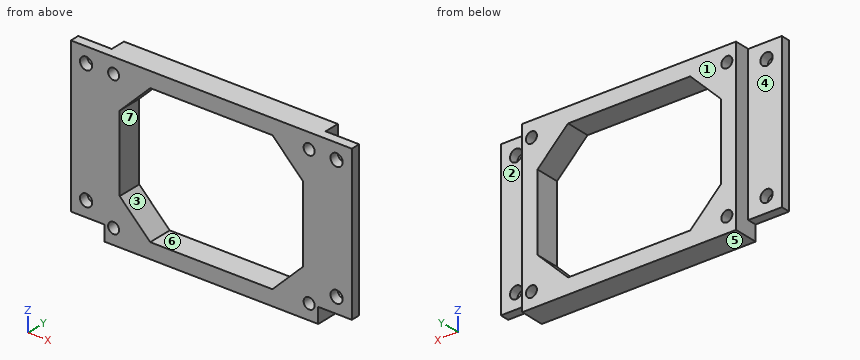
```python
from build123d import *

# Parameters (mm, degrees)
SKETCH1_W                = 70
SKETCH1_H                = 50
BOSS_EXTRUDE1_DEPTH      = 5
SKETCH2_W                = 92
SKETCH2_H                = 50
BOSS_EXTRUDE2_DEPTH      = 3
M3_CLEARANCE_HOLE1_D     = 4
M3_CLEARANCE_HOLE1_DEPTH = 10
M3_CLEARANCE_HOLE1_TIP   = 1.201721238
SKETCH9_W                = 70
SKETCH9_H                = 8
BOSS_EXTRUDE3_DEPTH      = 5
M3_CLEARANCE_HOLE3_D     = 3.6
M3_CLEARANCE_HOLE3_DEPTH = 10
M3_CLEARANCE_HOLE3_TIP   = 1.081549114
CUT_EXTRUDE1_DEPTH       = 56.497747702


with BuildPart() as part:
    # Sketch1 → Boss-Extrude1 (new body)
    with BuildSketch(Plane(origin=(0, 0, 0), x_dir=(1, 0, 0), z_dir=(0, 1, 0))):
        Rectangle(SKETCH1_W, SKETCH1_H)
    extrude(amount=BOSS_EXTRUDE1_DEPTH)

    # Sketch2 → Boss-Extrude2 (add)
    with BuildSketch(Plane.XZ):
        Rectangle(SKETCH2_W, SKETCH2_H)
    extrude(amount=BOSS_EXTRUDE2_DEPTH)

    # M3 Clearance Hole1
    with Locations(Plane(origin=(0, 0, 0), x_dir=(1, 0, 0), z_dir=(0, 1, 0))):
        with Locations((-41, 20), (-41, -20), (41, 20), (41, -20)):
            Hole(M3_CLEARANCE_HOLE1_D / 2, depth=M3_CLEARANCE_HOLE1_DEPTH)
            with Locations((0, 0, -(M3_CLEARANCE_HOLE1_DEPTH + M3_CLEARANCE_HOLE1_TIP / 2))):  # 118° drill point
                Cone(0, M3_CLEARANCE_HOLE1_D / 2, M3_CLEARANCE_HOLE1_TIP, mode=Mode.SUBTRACT)

    # Sketch9 → Boss-Extrude3 (add)
    with BuildSketch(Plane(origin=(0, 0, -25), x_dir=(-1, 0, 0), z_dir=(0, 0, -1))):
        with Locations((0, 1)):
            Rectangle(SKETCH9_W, SKETCH9_H)
    extrude(amount=BOSS_EXTRUDE3_DEPTH)

    # M3 Clearance Hole3
    with Locations(Plane(origin=(0, 5, 0), x_dir=(1, 0, 0), z_dir=(0, 1, 0))):
        with Locations((32, -20), (-32, 25), (32, 25), (-32, -20)):
            Hole(M3_CLEARANCE_HOLE3_D / 2, depth=M3_CLEARANCE_HOLE3_DEPTH)
            with Locations((0, 0, -(M3_CLEARANCE_HOLE3_DEPTH + M3_CLEARANCE_HOLE3_TIP / 2))):  # 118° drill point
                Cone(0, M3_CLEARANCE_HOLE3_D / 2, M3_CLEARANCE_HOLE3_TIP, mode=Mode.SUBTRACT)

    # Sketch12 → Cut-Extrude1 (cut, through all)
    with BuildSketch(Plane(origin=(0, 5, 0), x_dir=(1, 0, 0), z_dir=(0, 1, 0))):
        Polygon((20, -20), (30, -10), (30, 15), (20, 25), (-20, 25), (-30, 15), (-30, -10), (-20, -20), align=None)
    extrude(amount=-CUT_EXTRUDE1_DEPTH, mode=Mode.SUBTRACT)


solid = part.part
```
Build history of the part. All positions in model axes, mm. Face numbers are marked on the shaded views. A direction names the side the tool comes from. Give positions to 0.01 mm unless a question says otherwise; leave off trailing zeros. Order: outer loops, then holes, each group sorted by start corner. A loop starts at its lowest first (then second) coordinate and runs counter-clockwise, first axis right, second up. Notation, with made-up numbers: M 9,33.5 L 35,33.5 A8 cw 35,48.5 Z; hole C 36.5,-40 d1. An arc over 180 degrees is marked long. Return JSON: item names as keys, results as strings.
Q1. Band-saw the part on D-D (x = 41). Give the cut face in (y, z), then the cut area to 3 significant figures.
Answer list:
{"outline": "M -3,-25 L 0,-25 L 0,-22 L -3,-22 Z; M -3,-18 L 0,-18 L 0,18 L -3,18 Z; M -3,22 L 0,22 L 0,25 L -3,25 Z", "area": "126 mm^2"}
Q2. Band-saw the part on B-B (y = 2.25). Give the cut face in (x, z), then the cut area to 3 significant figures.
Answer list:
{"outline": "M -35,-30 L 35,-30 L 35,25 L -35,25 Z; hole C -32,-25 d3.6; hole C -32,20 d3.6; hole M -30,-15 L -20,-25 L 20,-25 L 30,-15 L 30,10 L 20,20 L -20,20 L -30,10 Z; hole C 32,-25 d3.6; hole C 32,20 d3.6", "area": "1,310 mm^2"}
Q3. 3-axis set-ups, long thin cutter, end or side, ignore diameter. For the marked faces 1, 2 and 3: which of +Z, -Z, +X, -X, +Y, -Y reach the whole face in a straight line?
Answer list:
{"face 1": "+Z, -Z, +X, -X, +Y", "face 2": "+Z, -Z, +X, +Y", "face 3": "+Y, -Y"}
Q4. Wall check: probe 1 along Z at (x, y) = (41, -1.5); probe 2 along X at (y, z) = (-0.25, -20); probe 3 along Z at (x, y) = (-32, 0.5). Give the ranges that are in metal, low to high. Write a range as from..to.
Answer list:
{"probe 1": "z = -25..-22, -18..18, 22..25", "probe 2": "x = -46..-43, -39..-25, 25..39, 43..46", "probe 3": "z = -30..-26.8, -23.2..18.2, 21.8..25"}
Q5. Band-saw the part on A-A (x = -27). Give the cut face in (y, z), then the cut area to 3 significant figures.
Answer list:
{"outline": "M -3,-30 L 5,-30 L 5,-18 L -3,-18 Z; M -3,13 L 5,13 L 5,25 L -3,25 Z", "area": "192 mm^2"}
Q6. Two-plate mould, pull along Z, no slides. Class the marked faces 4, 5, 6 and 7: pulls with the +Z half, pulls with the -Z half, needs draft (parallel to the pull), parting line crosses it, or undercut.
Answer list:
{"face 4": "needs draft", "face 5": "pulls with the -Z half", "face 6": "undercut", "face 7": "undercut"}
Q7. Band-saw the part on C-C (z = -8). Give the cut face in (x, y).
Answer list:
{"outline": "M -46,-3 L -30,-3 L -30,5 L -35,5 L -35,0 L -46,0 Z; M 30,-3 L 46,-3 L 46,0 L 35,0 L 35,5 L 30,5 Z"}
Q8. Flat gauge pins, fed straight in: pin 1 (3.5 mm diameter, centred on x = -41, z = -20, fed in from -Y); pin 2 (2.5 mm diameter, centred on y = 2.5, z = -9, fed in from -X); pin 3 (3.5 mm diameter, centred on x = -41, y = -1.5, fed in from -Z); pin 4 (9 mm diameter, centred on x = -43, z = -12.5, fed in from +Y). Where does each tip first touch, or does it go through?
Answer list:
{"pin 1": "passes through", "pin 2": "stops at x = -35", "pin 3": "stops at z = -25", "pin 4": "stops at y = 0"}
